```python
from build123d import *

# Parameters (mm, degrees)
SKETCH_1_R          = 20
SKETCH_1_R_2        = 10
EXTRUDE_1_DEPTH     = 60
EXTRUDE_2_DEPTH     = 30
SKETCH_4_R          = 10
EXTRUDE_3_DEPTH     = 10
SKETCH_8_R          = 10
CUT_EXTRUDE_1_DEPTH = 100
FILLET_1_R          = 50
FILLET_2_R          = 3


with BuildPart() as part:
    # 草图1 → 凸台-拉伸1 (new body)
    with BuildSketch(Plane.XY):
        Circle(SKETCH_1_R)
        Circle(SKETCH_1_R_2, mode=Mode.SUBTRACT)
    extrude(amount=EXTRUDE_1_DEPTH)

    # 草图2 → 凸台-拉伸2 (add, symmetric)
    with BuildSketch(Plane.XY.offset(30)):
        with BuildLine():
            Line((-14.142135624, 14.142135624), (-90, -61.715728753))
            Line((-90, -61.715728753), (-90, -320))
            Line((-90, -320), (-50, -320))
            Line((-50, -320), (-50, -78.284271247))
            Line((-50, -78.284271247), (14.142135624, -14.142135624))
            ThreePointArc((14.142135624, -14.142135624), (-14.142135624, -14.142135624), (-14.142135624, 14.142135624))
        make_face()
    extrude(amount=EXTRUDE_2_DEPTH, both=True)

    # 草图4 → 凸台-拉伸3 (add)
    with BuildSketch(Plane.XY.offset(60)):
        with BuildLine():
            Line((-90, -290), (-50, -290))
            Line((-50, -290), (-50, -350))
            ThreePointArc((-50, -350), (-70, -370), (-90, -350))
            Line((-90, -350), (-90, -290))
        make_face()
        with Locations((-70, -350)):
            Circle(SKETCH_4_R, mode=Mode.SUBTRACT)
    extrude_3 = extrude(amount=EXTRUDE_3_DEPTH)

    # 镜向1: 凸台-拉伸3 across plane
    add(extrude_3.mirror(Plane.XY.offset(30)))

    # 草图8 → 切除-拉伸1 (cut)
    with BuildSketch(Plane.XY.offset(60)):
        with Locations((-35.355339059, -35.355339059)):
            Circle(SKETCH_8_R)
    extrude(amount=-CUT_EXTRUDE_1_DEPTH, mode=Mode.SUBTRACT)

    # 圆角1
    fillet_1_edges = [part.edges().sort_by_distance(p)[0] for p in [
        (-50, -78.284271247, 30),
        (-90, -61.715728753, 30),
    ]]
    fillet(fillet_1_edges, radius=FILLET_1_R)

    # 圆角2
    fillet_2_edges = [part.edges().sort_by_distance(p)[0] for p in [
        (14.142135624, 14.142135624, 60),
        (14.142135624, 14.142135624, 0),
        (-10.606601718, -38.890872965, 60),
        (-44.748737342, -16.464466094, 0),
        (-70, -320, 0),
        (-90, -320, 30),
        (-50, -320, 30),
        (-44.748737342, -16.464466094, 60),
        (-70, -320, 60),
        (-10.606601718, -38.890872965, 0),
        (-90, -320, 70),
        (-70, -370, 70),
        (-50, -320, 70),
        (-70, -290, 70),
        (-90, -335, 60),
        (-90, -290, 65),
        (-70, -370, 60),
        (-50, -335, 60),
        (-90, -320, -10),
        (-70, -290, -10),
        (-90, -290, -5),
        (-50, -320, -10),
        (-70, -370, -10),
        (-90, -335, 0),
        (-70, -370, 0),
        (-50, -335, 0),
        (-90, -186.213203436, 0),
        (-90, -186.213203436, 60),
        (-50, -194.497474683, 0),
        (-86.193976626, -63.292235253, 0),
        (-50, -194.497474683, 60),
        (-86.193976626, -63.292235253, 60),
        (-46.193976626, -79.860777748, 0),
        (-46.193976626, -79.860777748, 60),
    ]]
    fillet(fillet_2_edges, radius=FILLET_2_R)


solid = part.part
```
Read the model definition and answer for the solid it produces. Units are mm, in the model's axes. A direction names the side the tool comes from. Coordinates: 2 decimals unless noted, no trailing zeros. Loops run counter-clockwise (first coordinate to the right, second up) from the corner with the lowest first, then second, coordinate; pieces in that order, holes last.
(1) The part is cut by section B-B (z = 25.5). Determine the outline of the cut face in (x, y).
Solution:
outline: (-90, -317) arc R3 ccw to (-87, -320) - (-53, -320) arc R3 ccw to (-50, -317) - (-50, -98.99) arc R50 cw to (-35.36, -63.64) - (14.14, -14.14) arc R20 ccw to (-14.14, 14.14) - (-75.36, -47.07) arc R50 ccw to (-90, -82.43) - close; hole circle Ø20 at (-35.36, -35.36); hole circle Ø20 at (0, 0)
(2) Flat-ended cylindrical pins translate along their axes: pin 1 Ø10 at (x, y) = (-73, -347) entering from +Z; pin 2 Ø5 at (x, z) = (-75.5, -4) entering from +Y; pin 3 Ø8 at (y, z) = (-296.5, 6.5) entering from +X; pin 4 Ø3 at (x, z) = (-72.5, 2.5) entering from +Y. Find the tip coordinate at first contact, or state that the pin passes through.
Solution:
pin 1: passes through
pin 2: stops at y = -290
pin 3: stops at x = -50
pin 4: stops at y = -42.75
(3) A tool of negligible diameter and unlimited length cuts with its end or side. For faces 5 (the face through (-50, -223, 31)), 6 (the face through (-71.302, -340.085, 64.93)), 7 (the face through (-58, -147, 60)), 8 (the face through (-69.8, -339.8, 0)), from which of +Z, -Z, +X, -X, +Y, -Y can it reach the whole face along a straight path? Write none if from no direction.
Solution:
face 5: +Z, -Z, +X, -Y
face 6: +Z, -Z
face 7: +Z, +X, -X, +Y
face 8: +X, -X, -Y
(4) Consider line 1 along Y through (x, z) = (-70, 67.25); line 2 along X through (y, z) = (-213, 17.5); line 3 along Z through (x, y) = (-74, -272). Determine where each line is inside the solid, lowest interval first.
Solution:
line 1: y = -369.99 to -360, -340 to -290.01
line 2: x = -90 to -50
line 3: z = 0 to 60
(5) The part is cut by section A-A (y = -261). Determine the outline of the cut face in (x, z), and give its area (3 significant figures).
Solution:
outline: (-90, 3) arc R3 ccw to (-87, 0) - (-53, 0) arc R3 ccw to (-50, 3) - (-50, 57) arc R3 ccw to (-53, 60) - (-87, 60) arc R3 ccw to (-90, 57) - close
area: 2,390 mm2
(6) The mould has two halves that part along Y. Classify faces 1 (the face through (-44.539, -17.531, 0.855)), 2 (the face through (-70, -329, 70)), 3 (the face through (-71.302, -340.085, -4.93)), 4 (the face through (-70, -320, 30)): released by +Y, released by -Y, zero draft, split by the parting line, or undercut.
Solution:
face 1: released by +Y
face 2: zero draft
face 3: undercut
face 4: released by -Y
